Geometry: final body of the model. Coordinates: model frame, mm. A direction names the side the tool comes from. Give positions to 0.01 mm unless a question says otherwise; leave off trailing zeros. Order: outer loops, then holes, each group sorted by start corner. A loop starts at its lowest first (then second) coordinate and runs counter-clockwise, first axis right, second up. Notation, with made-up numbers: (-32.5, 73.5) -> (-13.5, 73.5) arc R28 ccw to (-13.5, 97.5) -> close; hole circle Ø7 at (67.5, 24.25). An arc over 180 degrees is marked (long way). One line per question, with ' | ' between items.
from build123d import *

# Parameters (mm, degrees)
SKETCH_W         = 37
SKETCH_H         = 63
PAD_DEPTH        = 17.5
SKETCH001_W      = 32.7
SKETCH001_H      = 59.2
POCKET_DEPTH     = 15.6
SKETCH002_R      = 2
PAD001_DEPTH     = 1
FILLET_R         = 0.9
FILLET001_R      = 0.9
SKETCH004_W      = 3
SKETCH004_H      = 13.390789
POCKET001_DEPTH  = 5
FILLET002_R      = 1
SKETCH005_W      = 3.455711
SKETCH005_H      = 3.543194
REVOLUTION_ANGLE = 180
FILLET003_R      = 1


with BuildPart() as part:
    # Sketch → Pad (new body)
    with BuildSketch(Plane.XY):
        with Locations((18.5, -31.5)):
            Rectangle(SKETCH_W, SKETCH_H)
    extrude(amount=PAD_DEPTH)

    # Sketch001 (on Face6 of Pad) → Pocket (cut)
    with BuildSketch(Plane.XY.offset(17.5)):
        with Locations((18.35, -31.5)):
            Rectangle(SKETCH001_W, SKETCH001_H)
    extrude(amount=-POCKET_DEPTH, mode=Mode.SUBTRACT)

    # Sketch002 (on Face10 of Pocket) → Pad001 (join)
    with BuildSketch(Plane.XZ.offset(1.9)):
        with Locations((11, 9)):
            Circle(SKETCH002_R)
        with Locations((25.5, 9)):
            Circle(SKETCH002_R)
    extrude(amount=PAD001_DEPTH)

    # Fillet
    fillet_edges = [part.edges().sort_by_distance(p)[0] for p in [
        (9, -2.9, 9),
    ]]
    fillet(fillet_edges, radius=FILLET_R)

    # Fillet001
    fillet001_edges = [part.edges().sort_by_distance(p)[0] for p in [
        (23.5, -2.9, 9),
    ]]
    fillet(fillet001_edges, radius=FILLET001_R)

    # Sketch004 (on Face11 of Fillet001) → Pocket001 (cut)
    with BuildSketch(Plane(origin=(0, 0, 0), x_dir=(-1, 0, 0), z_dir=(0, 1, 0))):
        with Locations((-18.5, 20.695394)):
            Rectangle(SKETCH004_W, SKETCH004_H)
    extrude(amount=-POCKET001_DEPTH, mode=Mode.SUBTRACT)

    # Fillet002
    fillet002_edges = [part.edges().sort_by_distance(p)[0] for p in [
        (18.5, 0, 0),
        (18.35, -61.1, 1.9),
        (13, -1.95, 9),
        (37, 0, 8.75),
        (9, -2, 9),
        (2, -31.5, 1.9),
        (34.7, -31.5, 1.9),
        (2, -61.1, 9.7),
        (37, -31.5, 0),
        (0, -31.5, 0),
        (18.5, -63, 0),
        (0, -63, 8.75),
        (37, -63, 8.75),
        (0, 0, 8.75),
    ]]
    fillet(fillet002_edges, radius=FILLET002_R)

    # Sketch005 (on Face15 of Fillet002) → Revolution (revolve)
    with BuildSketch(Plane(origin=(0, 0, 0), x_dir=(-1, 0, 0), z_dir=(0, 1, 0))):
        with Locations((-2.781869, 15.6677)):
            Rectangle(SKETCH005_W, SKETCH005_H)
    revolve(axis=Axis((18.5, 0, 22.777559), (0, 0, -1)), revolution_arc=REVOLUTION_ANGLE)

    # Fillet003
    fillet003_edges = [part.edges().sort_by_distance(p)[0] for p in [
        (17, -0.95, 14),
        (20, -0.95, 14),
    ]]
    fillet(fillet003_edges, radius=FILLET003_R)


solid = part.part
1) Contact query for flat-ended pins moving along their axis: pin 1 Ø5 at (x, z) = (11.5, 8.5) entering from +Y; pin 2 Ø5 at (x, y) = (27, -6) entering from +Z; pin 3 Ø1.1 at (x, y) = (18.5, -0.5) entering from +Z. Output: stop coordinate, or through.
Check result:
pin 1: stops at y = 0 | pin 2: stops at z = 1.9 | pin 3: stops at z = 14
2) Pull-direction query (X, two-part tool) for faces 6 (the flat face through (18, 15, 13.896)), 7 (the cylindrical face through (18.12, 17.44, 15.69)), 8 (the flat face through (2, -31, 10)); classes: +X half, -X half, draft (parallel to the pull), parting line (faces both ways), or undercut.
Check result:
face 6: draft | face 7: parting line | face 8: undercut
3) Section D-D on y = -11.5. Return loops of the section in (x, z).
Check result:
outline: (0, 1) arc R1 ccw to (1, 0) -> (36, 0) arc R1 ccw to (37, 1) -> (37, 17.5) -> (34.7, 17.5) -> (34.7, 2.9) arc R1 cw to (33.7, 1.9) -> (3, 1.9) arc R1 cw to (2, 2.9) -> (2, 17.5) -> (0, 17.5) -> close
4) Set-up query: faces 1 (the flat face through (18, 0, 9)), 2 (the flat face through (20, -1, 16)), 3 (the flat face through (37, -32, 9)), 4 (the cylindrical face through (18.192, 13.987, 15.693)), 5 (the flat face through (18, 15, 17.439)). Return all of +Z, -Z, +X, -X, +Y, -Y with unobstructed straight access to the full face (end or side cutting, diameter ignored); none if empty.
Check result:
face 1: -Z | face 2: +Z | face 3: +Z, -Z, +X, +Y, -Y | face 4: +Z, -Z | face 5: +Z, +X, -X, +Y
5) Material intervals for probe 1 along Y at (x, z) = (17, 13); probe 2 along X at (y, z) = (-27.5, 5.75); probe 3 along Z at (x, y) = (15.5, -20.5), sorted ascending. Write a range as from..to.
Check result:
probe 1: y = -63..-61.1, -1.9..0 | probe 2: x = 0..2, 34.7..37 | probe 3: z = 0..1.9
6) Section A-A on x = 22.5. Return loops of the section in (y, z), plus the area to 3 significant figures.
Check result:
outline: (-63, 1) arc R1 ccw to (-62, 0) -> (-1, 0) arc R1 ccw to (0, 1) -> (0, 17.5) -> (-1.9, 17.5) -> (-1.9, 1.9) -> (-60.1, 1.9) arc R1 cw to (-61.1, 2.9) -> (-61.1, 17.5) -> (-63, 17.5) -> close; (13.41, 13.9) -> (16.98, 13.9) -> (16.98, 17.44) -> (13.41, 17.44) -> close | area: 191 mm^2
7) Section C-C on y = 7.5. Return loops of the section in (x, z), plus the area to 3 significant figures.
Check result:
outline: (2.75, 13.9) -> (6.69, 13.9) -> (6.69, 17.44) -> (2.75, 17.44) -> close; (30.31, 13.9) -> (34.25, 13.9) -> (34.25, 17.44) -> (30.31, 17.44) -> close | area: 27.9 mm^2
8) Section B-B on z = 12.25. Return loops of the section in (x, y), plus the area to 3 significant figures.
Check result:
outline: (0, -62) arc R1 ccw to (1, -63) -> (36, -63) arc R1 ccw to (37, -62) -> (37, -1) arc R1 ccw to (36, 0) -> (1, 0) arc R1 ccw to (0, -1) -> close; hole (2, -60.1) arc R1 ccw to (3, -61.1) -> (34.7, -61.1) -> (34.7, -1.9) -> (2, -1.9) -> close | area: 395 mm^2
